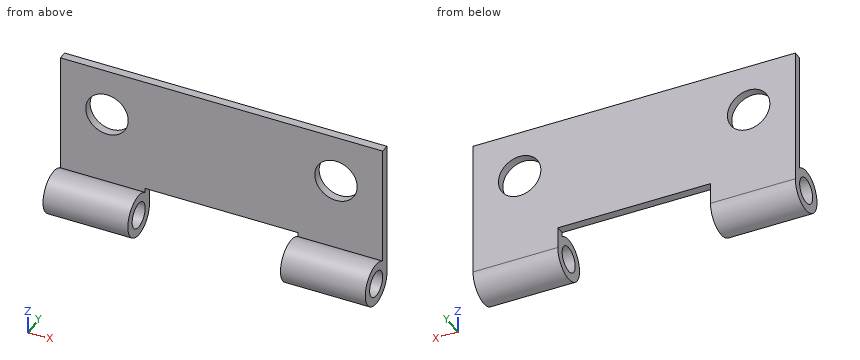
```python
from build123d import *

# Parameters (mm, degrees)
SKETCH3_R           = 1.5
BOSS_EXTRUDE2_DEPTH = 38
SKETCH6_W           = 18
SKETCH6_H           = 5
CUT_EXTRUDE1_DEPTH  = 6
SKETCH7_R           = 2.5
CUT_EXTRUDE2_DEPTH  = 10


with BuildPart() as part:
    # Sketch3 → Boss-Extrude2 (new body)
    with BuildSketch(Plane(origin=(0, 0, 0), x_dir=(0, 0, -1), z_dir=(1, 0, 0))):
        with BuildLine():
            Line((16, 1), (0, 1))
            Line((0, 1), (0, 0))
            Line((0, 0), (14, 0))
            ThreePointArc((14, 0), (17.118033989, -3.736067977), (16, 1))
        make_face()
        with Locations((16, -1.5)):
            Circle(SKETCH3_R, mode=Mode.SUBTRACT)
    extrude(amount=BOSS_EXTRUDE2_DEPTH)

    # Sketch6 → Cut-Extrude1 (cut, through all)
    with BuildSketch(Plane(origin=(0, 1, 0), x_dir=(1, 0, 0), z_dir=(0, 1, 0))):
        with Locations((19, 16)):
            Rectangle(SKETCH6_W, SKETCH6_H)
    extrude(amount=-CUT_EXTRUDE1_DEPTH, mode=Mode.SUBTRACT)

    # Sketch7 → Cut-Extrude2 (cut)
    with BuildSketch(Plane(origin=(0, 1, 0), x_dir=(1, 0, 0), z_dir=(0, 1, 0))):
        with Locations((5.5, 5.5)):
            Circle(SKETCH7_R)
        with Locations((32.5, 5.5)):
            Circle(SKETCH7_R)
    extrude(amount=-CUT_EXTRUDE2_DEPTH, mode=Mode.SUBTRACT)


solid = part.part
```
Check sheet for the modelled part. Datum: model origin and axes. Units: mm. Coordinates: 2 decimals unless noted, no trailing zeros. Loops run counter-clockwise (first coordinate to the right, second up) from the corner with the lowest first, then second, coordinate; pieces in that order, holes last.
1) Material ranges on probe 1 along X at (y, z) = (0.25, -5.5); probe 2 along Z at (x, y) = (34, -1.5); probe 3 along X at (y, z) = (-1.4, -14), recorded low to high.
2) Sectioned sample at C-C (y = -1.5). Record the boundary of the cut face in (x, z).
3) Sectioned sample at D-D (x = 35.5). Record the boundary of the cut face in (y, z).
4) Gauge pin test, flat ends, axial feed: pin 1 (4.5 mm diameter, centred on x = 5.5, z = -5.5, fed in from -Y); pin 2 (11 mm diameter, centred on x = 19.5, z = -4, fed in from -Y); pin 3 (0.8 mm diameter, centred on x = 22, y = 0.5, fed in from -Z). Record the tip position at first contact, or that the pin passes through.
5) Sectioned sample at B-B (z = -5.5). Record the boundary of the cut face in (x, y), and give its area (3 significant figures).
6) Sectioned sample at A-A (x = 5.5). Record the boundary of the cut face in (y, z), and give its area (3 significant figures).
Check sheet entries:
1. probe 1: x = 0 to 3, 8 to 30, 35 to 38
1. probe 2: z = -18.5 to -17.5, -14.5 to -13.5
1. probe 3: x = 0 to 10, 28 to 38
2. outline: (0, -18.5) - (10, -18.5) - (10, -17.5) - (0, -17.5) - close; (0, -14.5) - (10, -14.5) - (10, -13.5) - (0, -13.5) - close; (28, -18.5) - (38, -18.5) - (38, -17.5) - (28, -17.5) - close; (28, -14.5) - (38, -14.5) - (38, -13.5) - (28, -13.5) - close
3. outline: (0, -14) arc R2.5 ccw (long way) to (1, -16) - (1, 0) - (0, 0) - close; hole circle Ø3 at (-1.5, -16)
4. pin 1: passes through
4. pin 2: stops at y = 0
4. pin 3: stops at z = -13.5
5. outline: (0, 0) - (3, 0) - (3, 1) - (0, 1) - close; (8, 0) - (30, 0) - (30, 1) - (8, 1) - close; (35, 0) - (38, 0) - (38, 1) - (35, 1) - close
5. area: 28.0 mm2
6. outline: (0, -14) arc R2.5 ccw (long way) to (1, -16) - (1, -8) - (0, -8) - close; (0, -3) - (1, -3) - (1, 0) - (0, 0) - close; hole circle Ø3 at (-1.5, -16)
6. area: 22.2 mm2
